CAD build for the part. Positions are in the model's coordinates, mm. Coordinates: 2 decimals unless noted, no trailing zeros. Order: outer loops, then holes, each group sorted by start corner. A loop starts at its lowest first (then second) coordinate and runs counter-clockwise, first axis right, second up. Notation, with made-up numbers: (7, 88.25) - (43, 88.25) arc R20 ccw to (43, 94.25) - close; hole circle Ø10 at (-32.75, 63.25). An arc over 180 degrees is marked (long way). Write each question's results on one line, items separated by ' | '. Start each with the question number.
Q1. Wall check: probe 1 along Z at (x, y) = (2.25, 28); probe 2 along Z at (x, y) = (2.05, 4.63); probe 3 along Z at (x, y) = (3.6, 30). Give the ranges that are in metal, low to high.
Q2. Band-saw the part on C-C, the plane x = 1.55. Count the separate pieces of the cut face and the enclosed holes in it, then the cut area to 3 significant figures.
Q3. Pull direction Z, two halves, no side cores. Call faces 1 (the flat face through (2, 29, 127)), 2 (the flat face through (2, 29, 0)), 3 (the flat face through (4.394, 28, 63)), 4 (the cylindrical face through (2.166, 5.381, 22.984)): released by +Z, released by -Z, zero draft, split by the parting line, or undercut.
Q4. Band-saw the part on A-A, the plane y = 28.2. Write the cut outline in (x, z).
Q5. Pin check, flat tip, straight feed: P1, Ø6.5, axis at y = 31.75, z = 78.625, coming from the -X side. Stop position of the tip, or through.
Q6. Band-saw the part on B-B, the plane z = 67. Write the cut outline in (x, y), then the cut area to 3 significant figures.
```python
from build123d import *

# Parameters (mm, degrees)
SKETCH2_W           = 4.3942
SKETCH2_H           = 56.388
BOSS_EXTRUDE1_DEPTH = 127
SKETCH4_R           = 2.5
SKETCH4_R_2         = 2.413
SKETCH4_R_3         = 3.175
SKETCH4_R_4         = 4
CUT_EXTRUDE2_DEPTH  = 140.024873809


with BuildPart() as part:
    # Sketch2 → Boss-Extrude1 (new body)
    with BuildSketch(Plane.XY):
        with Locations((2.1971, 28.194)):
            Rectangle(SKETCH2_W, SKETCH2_H)
    extrude(amount=BOSS_EXTRUDE1_DEPTH)

    # Sketch4 → Cut-Extrude2 (cut, through all)
    with BuildSketch(Plane.ZY):
        with Locations((20.5994, 4.629999884)):
            Circle(SKETCH4_R)
        with Locations((9.525, 31.75)):
            Circle(SKETCH4_R_2)
        with Locations((67.7394, 4.629999884)):
            Circle(SKETCH4_R)
        with Locations((78.625, 31.75)):
            Circle(SKETCH4_R_2)
        with Locations((44.1706, 28.199999884)):
            Circle(SKETCH4_R_3)
        with Locations((94.9706, 28.199999884)):
            Circle(SKETCH4_R_4)
        with Locations((67.7394, 51.772399884)):
            Circle(SKETCH4_R)
        with Locations((20.5994, 51.772399884)):
            Circle(SKETCH4_R)
    extrude(amount=-CUT_EXTRUDE2_DEPTH, mode=Mode.SUBTRACT)


solid = part.part
```
Results below:
1) probe 1: z = 0 to 41, 47.34 to 90.98, 98.97 to 127 | probe 2: z = 0 to 18.1, 23.1 to 65.24, 70.24 to 127 | probe 3: z = 0 to 7.86, 11.19 to 41.56, 46.79 to 76.96, 80.29 to 91.4, 98.54 to 127
2) separate pieces: 1 | enclosed holes: 8 | area: 6,960 mm²
3) face 1: released by +Z | face 2: released by -Z | face 3: zero draft | face 4: undercut
4) outline: (0, 0) - (4.39, 0) - (4.39, 41) - (0, 41) - close; (0, 47.35) - (4.39, 47.35) - (4.39, 90.97) - (0, 90.97) - close; (0, 98.97) - (4.39, 98.97) - (4.39, 127) - (0, 127) - close
5) P1: stops at x = 0
6) outline: (0, 0) - (4.39, 0) - (4.39, 2.24) - (0, 2.24) - close; (0, 7.02) - (4.39, 7.02) - (4.39, 49.38) - (0, 49.38) - close; (0, 54.16) - (4.39, 54.16) - (4.39, 56.39) - (0, 56.39) - close | area: 206 mm²
